from build123d import *

# Parameters (mm, degrees)
F_01_START                          = -3
S01_LOW_FLANGED_HEAD_R              = 8
F_01_LOW_FLANGED_HEAD_DEPTH         = 3
S02_M5_THREAD_MAJOR_DIAMETER_R      = 2.5
F_02_M5_THREAD_MAJOR_DIAMETER_DEPTH = 8
F_03_START                          = -3.1
F_03_DRIVE_HEX_DEPTH                = 1.7


with BuildPart() as part:
    # S01 - Low flanged head → 01 - Low flanged head (new body)
    with BuildSketch(Plane.XY.offset(F_01_START)):
        Circle(S01_LOW_FLANGED_HEAD_R)
    extrude(amount=F_01_LOW_FLANGED_HEAD_DEPTH)

    # S02 - M5 thread major diameter → 02 - M5 thread major diameter (add)
    with BuildSketch(Plane.XY):
        Circle(S02_M5_THREAD_MAJOR_DIAMETER_R)
    extrude(amount=F_02_M5_THREAD_MAJOR_DIAMETER_DEPTH)

    # S03 - Drive hex → 03 - Drive hex (cut)
    with BuildSketch(Plane.XY.offset(F_03_START)):
        Polygon((1.732050808, 0), (0.866025404, 1.5), (-0.866025404, 1.5), (-1.732050808, 0), (-0.866025404, -1.5), (0.866025404, -1.5), align=None)
    extrude(amount=F_03_DRIVE_HEX_DEPTH, mode=Mode.SUBTRACT)


solid = part.part
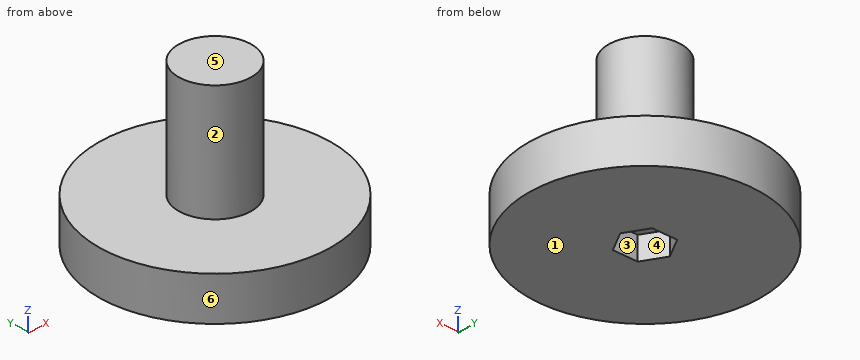
Geometry: final body of the model. Coordinates: model frame, mm. Face numbers are marked on the shaded views. A direction names the side the tool comes from. Round coordinates to 2 decimals unless told otherwise and drop trailing zeros. Order: outer loops, then holes, each group sorted by start corner. A loop starts at its lowest first (then second) coordinate and runs counter-clockwise, first axis right, second up. Notation, with made-up numbers: (-4, -2.5) - (46, -2.5) arc R16 cw to (46, 26.5) - close; hole circle Ø10 at (20.25, -8). An arc over 180 degrees is marked (long way). Write each question's results on one line, items separated by ' | '.
Item 1: Section A-A, the plane x = 0. Return the cut outline in (y, z), and give its area (3 significant figures).
Completed:
outline: (-8, -3) - (-1.5, -3) - (-1.5, -1.4) - (1.5, -1.4) - (1.5, -3) - (8, -3) - (8, 0) - (2.5, 0) - (2.5, 8) - (-2.5, 8) - (-2.5, 0) - (-8, 0) - close | area: 83.2 mm^2
Item 2: Material intervals for line 1 along Z through (x, y) = (-3.25, 6.5); line 2 along X through (y, z) = (-1.5, 3.5); line 3 along X through (y, z) = (-0.5, 2.5), sorted ascending. Write a range as [from, to].
Completed:
line 1: [-3, 0] | line 2: [-2, 2] | line 3: [-2.45, 2.45]
Item 3: First-contact query: pin 1 Ø1.5 at (x, z) = (0.5, 3) entering from +Y; pin 2 Ø4 at (x, z) = (3, 0.5) entering from -Y; pin 3 Ø5 at (x, z) = (2, 3) entering from -Y. Flat tips, straight axial feed; report the tip coordinate or a pass-through.
Completed:
pin 1: y = 2.5 | pin 2: y = -7.93 | pin 3: y = -2.5
Item 4: Section B-B, the plane z = 6. Return the cut outline in (x, y).
Completed:
outline: circle Ø5 at (0, 0)
Item 5: Section C-C, the plane y = 0.5. Return the cut outline in (x, z).
Completed:
outline: (-7.98, -3) - (-1.44, -3) - (-1.44, -1.4) - (1.44, -1.4) - (1.44, -3) - (7.98, -3) - (7.98, 0) - (2.45, 0) - (2.45, 8) - (-2.45, 8) - (-2.45, 0) - (-7.98, 0) - close
Item 6: Mould query, pull axis Y, two halves, no side actions, for the marked faces 4, 5 and 6. Classes: pulls with the +Y half, pulls with the -Y half, needs draft (parallel to the pull), parting line crosses it, or undercut.
Completed:
face 4: undercut | face 5: needs draft | face 6: parting line crosses it
Item 7: Reachability of the marked faces 1, 2 and 3 from +Z, -Z, +X, -X, +Y, -Y: full face, straight path, thin tool, end or side. Return the list, or none.
Completed:
face 1: -Z, +X, -X, +Y, -Y | face 2: +Z | face 3: -Z
Item 8: Section D-D, the plane x = -2.25. Return the cut outline in (y, z), and give its area (3 significant figures).
Completed:
outline: (-7.68, -3) - (7.68, -3) - (7.68, 0) - (1.09, 0) - (1.09, 8) - (-1.09, 8) - (-1.09, 0) - (-7.68, 0) - close | area: 63.5 mm^2
